```python
from build123d import *

# Parameters (mm, degrees)
F0_W     = 14.5
F0_H     = 7.5
F1_DEPTH = 0.8
F2_DEPTH = 93.6
F3_R     = 0.39999
F4_R     = 0.4
F5_W     = 18
F5_H     = 0.8
F6_W     = 18
F6_H     = 0.8
F7_DEPTH = 0.4
F8_R     = 0.39999


# Not quite as in the source:
# - a fillet or chamfer is up to 0.001 mm smaller than in the source, because OpenCascade refuses the exact size
# - a feature names something its author has since deleted; it is built from what else it names


with BuildPart() as f1:
    # F0 (on Top) → F1 (new body)
    with BuildSketch(Plane.XY):
        with BuildLine():
            Line((9, 12.55), (-9, 12.55))
            ThreePointArc((-9, 12.55), (-21.55, 0), (-9, -12.55))
            Line((-9, -12.55), (9, -12.55))
            ThreePointArc((9, -12.55), (21.55, 0), (9, 12.55))
        make_face()
        with BuildLine():
            ThreePointArc((-9, -11.75), (-20.75, 0), (-9, 11.75))
            Line((-9, 11.75), (9, 11.75))
            ThreePointArc((9, 11.75), (20.75, 0), (9, -11.75))
            Line((9, -11.75), (-9, -11.75))
        make_face(mode=Mode.SUBTRACT)
        with BuildLine():
            Line((9, 11.75), (-9, 11.75))
            ThreePointArc((-9, 11.75), (-20.75, 0), (-9, -11.75))
            Line((-9, -11.75), (9, -11.75))
            ThreePointArc((9, -11.75), (20.75, 0), (9, 11.75))
        make_face()
        with Locations((-7.25, 0)):
            Rectangle(F0_W, F0_H, mode=Mode.SUBTRACT)
    extrude(amount=F1_DEPTH)

    # F0 (on Top) → F2 (join)
    with BuildSketch(Plane.XY):
        with BuildLine():
            Line((9, 12.55), (-9, 12.55))
            ThreePointArc((-9, 12.55), (-21.55, 0), (-9, -12.55))
            Line((-9, -12.55), (9, -12.55))
            ThreePointArc((9, -12.55), (21.55, 0), (9, 12.55))
        make_face()
        with BuildLine():
            ThreePointArc((-9, -11.75), (-20.75, 0), (-9, 11.75))
            Line((-9, 11.75), (9, 11.75))
            ThreePointArc((9, 11.75), (20.75, 0), (9, -11.75))
            Line((9, -11.75), (-9, -11.75))
        make_face(mode=Mode.SUBTRACT)
    extrude(amount=F2_DEPTH)

    # F3 (radius 0.4 in the source; OpenCascade refuses exactly that, so slightly less here)
    f3_edges = [f1.edges().sort_by_distance(p)[0] for p in [
        (0, -12.55, 93.6),
        (0, -11.75, 93.6),
        (0, -12.55, 0),
        (-7.25, 3.75, 0),
        (-7.25, 3.75, 0.8),
        (-14.5, 0, 0),
        (-14.5, 0, 0.8),
        (-7.25, -3.75, 0),
        (-7.25, -3.75, 0.8),
        (0, 0, 0),
        (0, 0, 0.8),
    ]]
    fillet(f3_edges, radius=F3_R)

    # F4
    f4_edges = [f1.edges().sort_by_distance(p)[0] for p in [
        (0, 11.75, 0.8),
    ]]
    fillet(f4_edges, radius=F4_R)

    # F5 (on face) + F6 (on face) → F7 (join, symmetric)
    with BuildSketch(Plane.XZ.offset(-11.75)):
        with Locations((0, 92.8)):
            Rectangle(F5_W, F5_H)
    with BuildSketch(Plane(origin=(0, -11.75, 0), x_dir=(-1, 0, 0), z_dir=(0, 1, 0))):
        with Locations((0, 92.8)):
            Rectangle(F6_W, F6_H)
    extrude(amount=F7_DEPTH, both=True, dir=(0, -1, 0))

    # F8 (radius 0.4 in the source; OpenCascade refuses exactly that, so slightly less here)
    f8_edges = [f1.edges().sort_by_distance(p)[0] for p in [
        (0, 11.35, 93.2),
        (0, 11.35, 92.4),
        (-9, 11.35, 92.8),
        (9, 11.35, 92.8),
        (0, -11.35, 93.2),
        (0, -11.35, 92.4),
        (9, -11.35, 92.8),
        (-9, -11.35, 92.8),
    ]]
    fillet(f8_edges, radius=F8_R)


solid = f1.part
```
The model under review builds one solid part; all positions refer to its coordinate system, in mm. A direction names the side the tool comes from. Coordinates: 2 decimals unless noted, no trailing zeros. Write each loop counter-clockwise with the first axis right and the second up, starting at its lowest first coordinate (ties: lowest second). Pieces come first, ordered by that corner, then holes. Notation, with made-up numbers: (-7, -35.75) - (7, -35.75) arc R14 ccw to (7, -19.75) - close; hole circle Ø10 at (49.5, 17.5). An arc over 180 degrees is marked (long way). Answer in a Markdown table with one row per item. Add a question column.
Q1. Clearance check with flat-ended pins moving along their axes: pin 1 (8 mm diameter, centred on y = 7, z = 42.5, fed in from +X); pin 2 (6 mm diameter, centred on x = -13.5, z = 68, fed in from +Y); pin 3 (4 mm diameter, centred on x = 7.5, y = 8.5, fed in from +Z). State where each tip first meets the part, or that it passes through.
Q2. To check wall thickness, follow line 1 along X through (y, z) = (0.5, 26); line 2 along Y through (x, z) = (-0.5, 25.5). State the ranges of each line that lie inside material, in increasing order. Write a range as from..to.
Q3. For faces 4 (the face through (-20.747, -0.258, 46.556)), 5 (the face through (0, -12.55, 46)), 6 (the face through (0, 11.75, 46)), list the 3-axis set-ups (+Z, -Z, +X, -X, +Y, -Y) from which the entire face can be reached by the end or side of a thin tool; tool diameter is ignored.
Q4. Consider section B-B on z = 32.5. Give the boundary of the cut face in (x, y).
Q5. Draft analysis for pull direction Z (two halves, no side actions). For faces 1 (the face through (0, -11.75, 46)), 2 (the face through (4, 0, 0.8)), 3 (the face through (-21.547, 0.276, 46.15)), state which applies: +Z half, -Z half, draft (parallel to the pull), parting line (faces both ways), or undercut.
Answers below:
| question | item | result |
|---|---|---|
| 1 | pin 1 | x = 21.19 |
| 1 | pin 2 | y = 12.46 |
| 1 | pin 3 | z = 0.8 |
| 2 | line 1 | -21.54..-20.74, 20.74..21.54 |
| 2 | line 2 | -12.55..-11.75, 11.75..12.55 |
| 3 | face 4 | +Z |
| 3 | face 5 | +Z, -Z, +X, -X, -Y |
| 3 | face 6 | none |
| 4 | outline | (-9, -12.55) - (9, -12.55) arc R12.55 ccw to (9, 12.55) - (-9, 12.55) arc R12.55 ccw to start; hole (-9, -11.75) - (9, -11.75) arc R11.75 ccw to (9, 11.75) - (-9, 11.75) arc R11.75 ccw to start |
| 5 | face 1 | undercut |
| 5 | face 2 | +Z half |
| 5 | face 3 | draft |
